Model file for the job. Use its own axes, mm. Face numbers are marked on the shaded views. A direction names the side the tool comes from. Give positions to 0.01 mm unless a question says otherwise; leave off trailing zeros. Order: outer loops, then holes, each group sorted by start corner. A loop starts at its lowest first (then second) coordinate and runs counter-clockwise, first axis right, second up. Notation, with made-up numbers: M -7.75,-27 L 17.25,-27 A12 cw 17.25,-22 Z; hole C -34,47.25 d3. An arc over 180 degrees is marked long. Return JSON: item names as keys, results as strings. Group by question number.
1. Pin check, flat tips, straight feed: pin 1 (3 mm diameter, centred on x = 4, z = 3, fed in from +Y); pin 2 (2 mm diameter, centred on x = -14, y = 2.5, fed in from +Z); pin 3 (0.9 mm diameter, centred on y = 3, z = 7, fed in from -X). Stop position of each tip, or through.
2. Wall check: probe 1 along X at (y, z) = (2.2, 4); probe 2 along X at (y, z) = (1.85, -5.75); probe 3 along X at (y, z) = (3.5, -1.5). Give the ranges that are in metal, low to high. Write a range as [from, to].
3. Two-plate mould, pull along X, no slides. Class the marked faces 1, 2 and 3: released by +X, released by -X, zero draft, split by the parting line, or undercut.
4. Slice it at B-B on z = 0. List the corners of the cut face in (x, y), then the cut area to 3 significant figures.
5. Slice it at A-A on y = 2. List the corners of the cut face in (x, z).
6. Slice it at C-C on x = 4. List the corners of the cut face in (y, z).
7. 3-axis set-ups, long thin cutter, end or side, ignore diameter. For the marked faces 4, 5, 6, 7 and 8: which of +Z, -Z, +X, -X, +Y, -Y reach the whole face in a straight line?
8. Slice it at D-D on z = 4. List the corners of the cut face in (x, y).
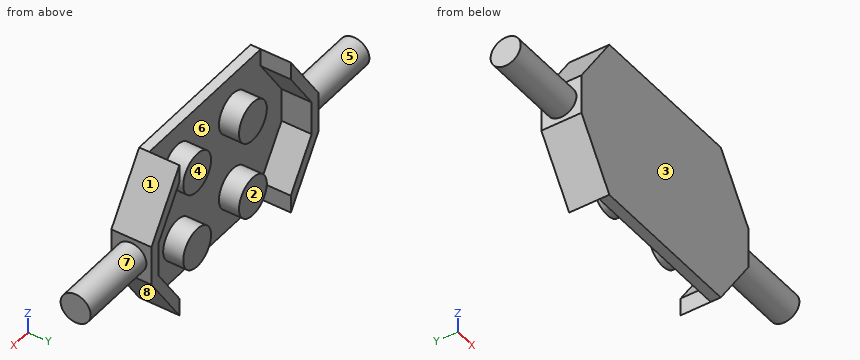
from build123d import *

# Parameters (mm, degrees)
BOSS_EXTRUDE1_DEPTH = 1
SKETCH2_R           = 2
BOSS_EXTRUDE2_DEPTH = 2
BOSS_EXTRUDE3_DEPTH = 3
SKETCH5_R           = 1.5
BOSS_EXTRUDE4_DEPTH = 8


with BuildPart() as part:
    # Sketch1 → Boss-Extrude1 (new body)
    with BuildSketch(Plane(origin=(0, 0, 0), x_dir=(1, 0, 0), z_dir=(0, 1, 0))):
        Polygon((0, -8), (0, 8), (-8, 8), (-12, 2), (-12, -2), (-8, -8), align=None)
    boss_extrude1 = extrude(amount=BOSS_EXTRUDE1_DEPTH)

    # Sketch2 → Boss-Extrude2 (add)
    with BuildSketch(Plane(origin=(0, 1, 0), x_dir=(1, 0, 0), z_dir=(0, 1, 0))):
        with Locations((-4, 4)):
            Circle(SKETCH2_R)
        with Locations((-4, -4)):
            Circle(SKETCH2_R)
    boss_extrude2 = extrude(amount=BOSS_EXTRUDE2_DEPTH)

    # Sketch3 → Boss-Extrude3 (add)
    with BuildSketch(Plane(origin=(0, 1, 0), x_dir=(1, 0, 0), z_dir=(0, 1, 0))):
        Polygon((-8, 6.197224362), (-11, 1.697224362), (-11, -1.697224362), (-8, -6.197224362), (-8, -8), (-12, -2), (-12, 2), (-8, 8), align=None)
    boss_extrude3 = extrude(amount=BOSS_EXTRUDE3_DEPTH)

    # Sketch5 → Boss-Extrude4 (add)
    with BuildSketch(Plane.ZY.offset(12)):
        with Locations((0, 2)):
            Circle(SKETCH5_R)
    boss_extrude4 = extrude(amount=BOSS_EXTRUDE4_DEPTH)

    # Mirror1: Boss-Extrude1, Boss-Extrude2, Boss-Extrude3, Boss-Extrude4 across plane
    add(boss_extrude1.mirror(Plane(origin=(0, 1, 8), x_dir=(0, 0, 1), z_dir=(-1, 0, 0))))
    add(boss_extrude2.mirror(Plane(origin=(0, 1, 8), x_dir=(0, 0, 1), z_dir=(-1, 0, 0))))
    add(boss_extrude3.mirror(Plane(origin=(0, 1, 8), x_dir=(0, 0, 1), z_dir=(-1, 0, 0))))
    add(boss_extrude4.mirror(Plane(origin=(0, 1, 8), x_dir=(0, 0, 1), z_dir=(-1, 0, 0))))


solid = part.part
Result:
{
 "1": {"pin 1": "stops at y = 3", "pin 2": "stops at z = 1.5", "pin 3": "stops at x = -8.97"},
 "2": {"probe 1": "x = [-10.67, -9.46], [-6, -2], [2, 6], [9.46, 10.67]", "probe 2": "x = [-9.5, -8.3], [-4.97, -3.03], [3.03, 4.97], [8.3, 9.5]", "probe 3": "x = [-12, -11], [11, 12]"},
 "3": {"face 1": "released by +X", "face 2": "undercut", "face 3": "zero draft"},
 "4": {"outline": "M -20,0.5 L -12,0.5 L -12,0 L 12,0 L 12,0.5 L 20,0.5 L 20,3.5 L 12,3.5 L 12,4 L 11,4 L 11,1 L -11,1 L -11,4 L -12,4 L -12,3.5 L -20,3.5 Z", "area": "78.0 mm2"},
 "5": {"outline": "M -20,-1.5 L -12,-1.5 L -12,-2 L -8,-8 L -8,-6.2 L -11,-1.7 L -11,1.7 L -8,6.2 L -8,8 L -12,2 L -12,1.5 L -20,1.5 Z; C -4,-4 d4; C -4,4 d4; C 4,-4 d4; C 4,4 d4; M 8,-8 L 12,-2 L 12,-1.5 L 20,-1.5 L 20,1.5 L 12,1.5 L 12,2 L 8,8 L 8,6.2 L 11,1.7 L 11,-1.7 L 8,-6.2 Z"},
 "6": {"outline": "M 0,-8 L 1,-8 L 1,-6 L 3,-6 L 3,-2 L 1,-2 L 1,2 L 3,2 L 3,6 L 1,6 L 1,8 L 0,8 Z"},
 "7": {"face 4": "+Z, -Z, +Y", "face 5": "-X", "face 6": "+Y", "face 7": "+X", "face 8": "-Z, +X, +Y, -Y"},
 "8": {"outline": "M -10.67,0 L 10.67,0 L 10.67,4 L 9.46,4 L 9.46,1 L 6,1 L 6,3 L 2,3 L 2,1 L -2,1 L -2,3 L -6,3 L -6,1 L -9.46,1 L -9.46,4 L -10.67,4 Z"}
}
